```python
from build123d import *

# Parameters (mm, degrees)
SKETCH2_R = 3


with BuildPart() as part:
    # Sweep1: sweep along a path in Sketch1
    with BuildLine(Plane(origin=(0, 0, 0), x_dir=(1, 0, 0), z_dir=(0, 1, 0))) as sweep1_path:
        Line((0, 0), (19, 0))
        ThreePointArc((19, 0), (23.242640687, -1.757359313), (25, -6))
        Line((25, -6), (25, -95))
    # Sketch2 → Sweep1 (sweep)
    with BuildSketch(Plane(origin=(0, 0, 0), x_dir=(0, 0, -1), z_dir=(1, 0, 0))):
        Circle(SKETCH2_R)
    sweep(path=sweep1_path.line)

    # Sketch3 → Revolve1 (revolve)
    with BuildSketch(Plane(origin=(0, 0, 0), x_dir=(1, 0, 0), z_dir=(0, 1, 0)), mode=Mode.PRIVATE) as revolve1_sk:
        Polygon((0, 0), (-15, 0), (0, -3), align=None)
    revolve(revolve1_sk.sketch.rotate(Axis((0, 0, 0), (-1, 0, 0)), 180), axis=Axis((0, 0, 0), (-1, 0, 0)))

    # Sketch4 → Revolve2 (revolve)
    with BuildSketch(Plane(origin=(0, 0, 0), x_dir=(1, 0, 0), z_dir=(0, 1, 0)), mode=Mode.PRIVATE) as revolve2_sk:
        Polygon((25, -95), (25, -110), (28, -95), align=None)
    revolve(revolve2_sk.sketch.rotate(Axis((25, 0, 95), (0, 0, 1)), 180), axis=Axis((25, 0, 95), (0, 0, 1)))


solid = part.part
```
Source: CAD feature listing. Evaluate the final solid. Frame: model axes, mm. A direction names the side the tool comes from. Round coordinates to 2 decimals unless told otherwise and drop trailing zeros. Loops run counter-clockwise (first coordinate to the right, second up) from the corner with the lowest first, then second, coordinate; pieces in that order, holes last.
(1) Section query B-B (x = 16). Output: boundary loops of the cut face in (y, z).
From the geometry:
outline: circle Ø6 at (0, 0)
(2) Access query for faces 1 (the cylindrical face through (10, 0, 3)), 2 (the cylindrical face through (22, 0, 51)). Directions: +Z, -Z, +X, -X, +Y, -Y. A direction counts if a zero-diameter tool reaches every point of the face in a straight line with its end or side. Return the directions, or none.
From the geometry:
face 1: -X
face 2: +Z
(3) Material intervals for probe 1 along X at (y, z) = (0.25, 83); probe 2 along Z at (x, y) = (12, -0.25); probe 3 along X at (y, z) = (1.5, 45), sorted ascending.
From the geometry:
probe 1: x = 22.01 to 27.99
probe 2: z = -2.99 to 2.99
probe 3: x = 22.4 to 27.6
(4) Section query A-A (z = 34). Output: boundary loops of the cut face in (x, y).
From the geometry:
outline: circle Ø6 at (25, 0)
(5) Contact query for flat-ended pins moving along their axis: pin 1 Ø3 at (x, y) = (18, 2) entering from -Z; pin 2 Ø1.5 at (y, z) = (1.5, 81.5) entering from -X; pin 3 Ø1 at (x, y) = (-9, 0) entering from +Z. Output: stop coordinate, or through.
From the geometry:
pin 1: stops at z = -2.96
pin 2: stops at x = 22.1
pin 3: stops at z = 1.3
